Work out the finished part from the listing and answer in its coordinate system (mm). A direction names the side the tool comes from. Give positions to 0.01 mm unless a question says otherwise; leave off trailing zeros. Order: outer loops, then holes, each group sorted by start corner. A loop starts at its lowest first (then second) coordinate and runs counter-clockwise, first axis right, second up. Notation, with made-up numbers: (75, 45) - (118, 45) arc R27 ccw to (118, 70) - close; hole circle Ø10 at (-29.5, 85.25). An arc over 180 degrees is marked (long way). Put each result on its own line as item: value.
```python
from build123d import *

# Parameters (mm, degrees)
SKETCH038_W     = 36.25
SKETCH038_H     = 10.5
PAD012_DEPTH    = 23
SKETCH039_R     = 1.65
POCKET026_DEPTH = 23.001
POCKET027_DEPTH = 20
CHAMFER014_SIZE = 1
CHAMFER015_SIZE = 1
CHAMFER016_SIZE = 2.5
CHAMFER017_SIZE = 0.4
CHAMFER018_SIZE = 0.4


with BuildPart() as part:
    # Sketch038 → Pad012 (new body)
    with BuildSketch(Plane.YZ):
        with Locations((18.125, 5.25)):
            Rectangle(SKETCH038_W, SKETCH038_H)
    extrude(amount=PAD012_DEPTH)

    # Sketch039 (on Face5 of Pad012) → Pocket026 (cut, through all)
    with BuildSketch(Plane(origin=(0, 0, 0), x_dir=(0, 1, 0), z_dir=(-1, 0, 0))):
        with Locations((4.5, -3.7)):
            Circle(SKETCH039_R)
        with Locations((31.75, -3.7)):
            Circle(SKETCH039_R)
    extrude(amount=-POCKET026_DEPTH, mode=Mode.SUBTRACT)

    # Sketch040 (on Face4 of Pocket026) → Pocket027 (cut)
    with BuildSketch(Plane(origin=(0, 0, 0), x_dir=(0, 1, 0), z_dir=(-1, 0, 0))):
        Polygon((10, -10.5), (10, -5.5), (15, -5.5), (15, -7), (11.5, -7), (11.5, -10.5), align=None)
        Polygon((24.75, -10.5), (24.75, -7), (21.25, -7), (21.25, -5.5), (26.25, -5.5), (26.25, -10.5), align=None)
    extrude(amount=-POCKET027_DEPTH, mode=Mode.SUBTRACT)

    # Chamfer014
    chamfer014_edges = [part.edges().sort_by_distance(p)[0] for p in [
        (0, 26.25, 8),
        (0, 23.75, 5.5),
        (0, 21.25, 6.25),
        (0, 23, 7),
        (0, 24.75, 8.75),
        (0, 15, 6.25),
        (0, 13.25, 7),
        (0, 12.5, 5.5),
        (0, 10, 8),
        (0, 11.5, 8.75),
    ]]
    chamfer(chamfer014_edges, length=CHAMFER014_SIZE)

    # Chamfer015
    chamfer015_edges = [part.edges().sort_by_distance(p)[0] for p in [
        (11.5, 36.25, 10.5),
        (11.5, 0, 10.5),
    ]]
    chamfer(chamfer015_edges, length=CHAMFER015_SIZE)

    # Chamfer016
    chamfer016_edges = [part.edges().sort_by_distance(p)[0] for p in [
        (11.5, 36.25, 0),
        (11.5, 0, 0),
    ]]
    chamfer(chamfer016_edges, length=CHAMFER016_SIZE)

    # Chamfer017
    chamfer017_edges = [part.edges().sort_by_distance(p)[0] for p in [
        (10.5, 26.25, 10.5),
        (0.5, 26.75, 10.5),
        (0.5, 24.25, 10.5),
        (10.5, 24.75, 10.5),
        (20, 25.5, 10.5),
        (20, 10.75, 10.5),
        (10.5, 11.5, 10.5),
        (0.5, 12, 10.5),
        (0.5, 9.5, 10.5),
        (10.5, 10, 10.5),
    ]]
    chamfer(chamfer017_edges, length=CHAMFER017_SIZE)

    # Chamfer018
    chamfer018_edges = [part.edges().sort_by_distance(p)[0] for p in [
        (23, 0, 6),
        (23, 1.25, 1.25),
        (23, 0.5, 10),
        (23, 18.125, 0),
        (23, 18.125, 10.5),
        (23, 35, 1.25),
        (23, 35.75, 10),
        (23, 36.25, 6),
        (23, 30.1, 3.7),
        (23, 2.85, 3.7),
    ]]
    chamfer(chamfer018_edges, length=CHAMFER018_SIZE)


with BuildPart() as part_1:
    # Body004006 placement: moved
    add(part.part.moved(Location((-66.5, -26, 6.5))))


solid = part_1.part
```
(1) Section B-B, the plane x = -54.25 is taken. Write down the section's boundary in (y, z).
Geometry check:
outline: (-26, 9) - (-23.5, 6.5) - (7.75, 6.5) - (10.25, 9) - (10.25, 16) - (9.25, 17) - (0.65, 17) - (0.25, 16.6) - (0.25, 12) - (-4.75, 12) - (-4.75, 13.5) - (-1.25, 13.5) - (-1.25, 16.6) - (-1.65, 17) - (-14.1, 17) - (-14.5, 16.6) - (-14.5, 13.5) - (-11, 13.5) - (-11, 12) - (-16, 12) - (-16, 16.6) - (-16.4, 17) - (-25, 17) - (-26, 16) - close; hole circle Ø3.3 at (-21.5, 10.2); hole circle Ø3.3 at (5.75, 10.2)
(2) Determine the mould class of faces 1 (the face through (-55.36, 9.02, 7.77)), 2 (the face through (-55, -8, 17)), 3 (the face through (-56, 0.25, 14)) for opening direction Y: pulls with the +Y half, pulls with the -Y half, needs draft (parallel to the pull), parting line crosses it, or undercut.
Geometry check:
face 1: pulls with the +Y half
face 2: needs draft
face 3: undercut
(3) Section D-D, the plane z = 15.25 is taken. Write down the section's boundary in (x, y), then the cut area to 3 significant figures.
Geometry check:
outline: (-66.5, -26) - (-43.9, -26) - (-43.5, -25.6) - (-43.5, 9.85) - (-43.9, 10.25) - (-66.5, 10.25) - (-66.5, 1.25) - (-65.5, 0.25) - (-46.5, 0.25) - (-46.5, -1.25) - (-65.5, -1.25) - (-66.5, -2.25) - (-66.5, -13.5) - (-65.5, -14.5) - (-46.5, -14.5) - (-46.5, -16) - (-65.5, -16) - (-66.5, -17) - close
area: 772 mm²
(4) Section A-A, the plane y = -21.5 is taken. Write down the section's boundary in (x, z).
Geometry check:
outline: (-66.5, 6.5) - (-43.9, 6.5) - (-43.5, 6.9) - (-43.5, 8.15) - (-43.9, 8.55) - (-66.5, 8.55) - close; (-66.5, 11.85) - (-43.9, 11.85) - (-43.5, 12.25) - (-43.5, 16.6) - (-43.9, 17) - (-66.5, 17) - close
(5) Straight lines are drawn through the part: line 1 (Y direction, x = -57.75, z = 10.2); line 2 (Y direction, x = -53, z = 13.25); line 3 (Z direction, x = -59.25, y = -21.5). For each, find the intervals that lie inside material, in ascending order.
Geometry check:
line 1: y = -26 to -23.15, -19.85 to 4.1, 7.4 to 10.25
line 2: y = -26 to -16, -11 to -4.75, 0.25 to 10.25
line 3: z = 6.5 to 8.55, 11.85 to 17
(6) A tool of negligible diameter and unlimited length cuts with its end or side. For faces 4 (the face through (-66.5, -8, 12)), 5 (the face through (-56, -3, 13.5)), 6 (the face through (-66.01, -2.04, 16.8)), from which of +Z, -Z, +X, -X, +Y, -Y can it reach the whole face along a straight path? Write none if from no direction.
Geometry check:
face 4: +Z, -Z, -X, +Y, -Y
face 5: -X
face 6: +Z, -X
(7) Section C-C, the plane z = 10.2 is taken. Write down the section's boundary in (x, y).
Geometry check:
outline: (-66.5, -26) - (-43.9, -26) - (-43.5, -25.6) - (-43.5, -23.55) - (-43.9, -23.15) - (-66.5, -23.15) - close; (-66.5, -19.85) - (-43.9, -19.85) - (-43.5, -19.45) - (-43.5, 3.7) - (-43.9, 4.1) - (-66.5, 4.1) - close; (-66.5, 7.4) - (-43.9, 7.4) - (-43.5, 7.8) - (-43.5, 9.85) - (-43.9, 10.25) - (-66.5, 10.25) - close
